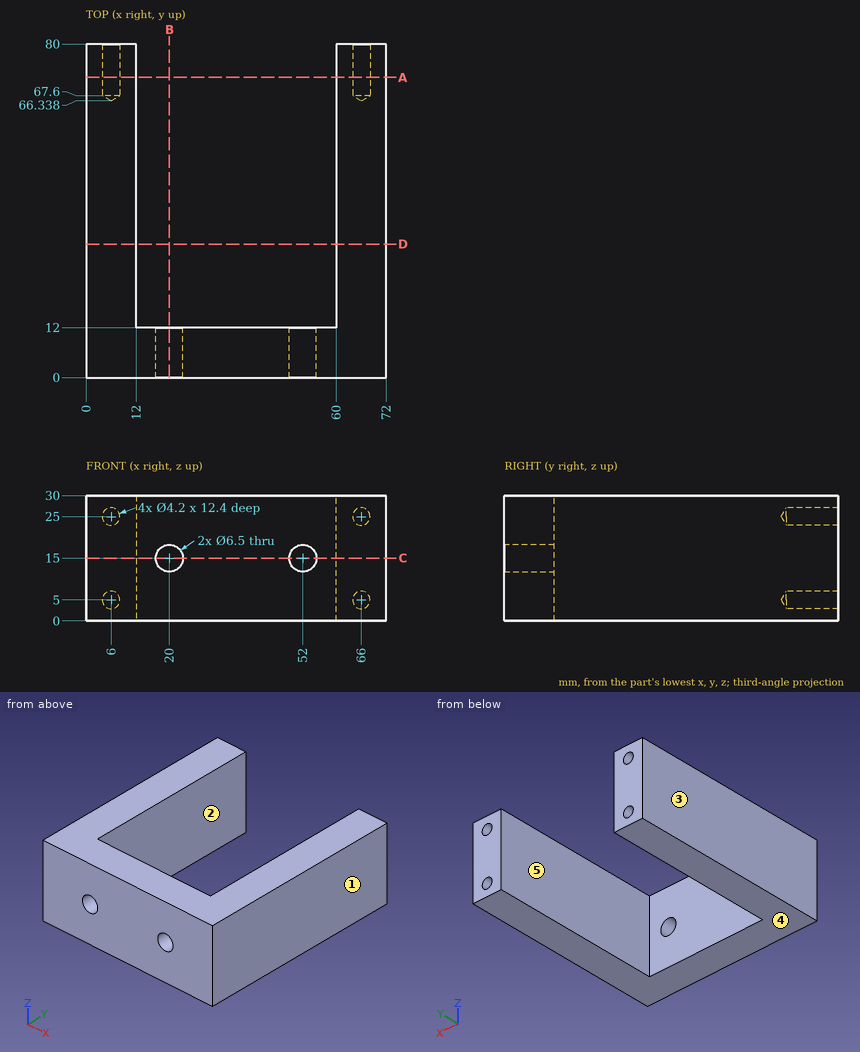
The drawing under review shows one solid part. Ordinate dimensions are in mm from its lowest x, y, z. A direction names the side the tool comes from. Coordinates: 2 decimals unless noted, no trailing zeros. Write each loop counter-clockwise with the first axis right and the second up, starting at its lowest first coordinate (ties: lowest second). Pieces come first, ordered by that corner, then holes. Notation, with made-up numbers: (-31.5, -14) - (11.5, -14) arc R30 cw to (11.5, 15) - close; hole circle Ø9 at (84.25, 38). An arc over 180 degrees is marked (long way). Answer as CSV lines item,"result".
(1) We need section A-A (y = 72). Give the boundary of the cut face in (x, z).
Data:
outline,"(0, 0) - (12, 0) - (12, 30) - (0, 30) - close; (60, 0) - (72, 0) - (72, 30) - (60, 30) - close; hole circle Ø4.2 at (6, 5); hole circle Ø4.2 at (6, 25); hole circle Ø4.2 at (66, 5); hole circle Ø4.2 at (66, 25)"
(2) We need section B-B (x = 20). Give the boundary of the cut face in (y, z).
Data:
outline,"(0, 0) - (12, 0) - (12, 11.75) - (0, 11.75) - close; (0, 18.25) - (12, 18.25) - (12, 30) - (0, 30) - close"
(3) Tool access review of the marked faces 1 and 2: name each direction out of +Z, -Z, +X, -X, +Y, -Y from which nothing blocks a thin tool from reaching the whole face with its end or side.
Data:
face 1,"+Z, -Z, +X, +Y, -Y"
face 2,"+Z, -Z, +Y"
(4) Mouldability with a two-part tool opening along X and no side actions: class the marked faces 3, 4 and 5 as pulls with the +X half, pulls with the -X half, needs draft (parallel to the pull), parting line crosses it, or undercut.
Data:
face 3,"pulls with the -X half"
face 4,"needs draft"
face 5,"undercut"
(5) We need section D-D (y = 32). Give the boundary of the cut face in (x, z).
Data:
outline,"(0, 0) - (12, 0) - (12, 30) - (0, 30) - close; (60, 0) - (72, 0) - (72, 30) - (60, 30) - close"
(6) Clearance check with flat-ended pins moving along their axes: pin 1 Ø2.5 at (x, z) = (6, 5) entering from +Y; pin 2 Ø4 at (x, z) = (21.5, 3.5) entering from +Y; pin 3 Ø4 at (x, z) = (52, 15) entering from +Y. State where each tip first meets the part, or that it passes through.
Data:
pin 1,"stops at y = 67.09"
pin 2,"stops at y = 12"
pin 3,"passes through"
(7) For line 1 along X through (y, z) = (6.25, 15); line 2 along X through (y, z) = (72, 5); line 3 along Z through (x, y) = (6, 71.25), list the stretches that pass through material, from the lowest coordinate up. Write a range as [from, to].
Data:
line 1,"x = [0, 16.75], [23.25, 48.75], [55.25, 72]"
line 2,"x = [0, 3.9], [8.1, 12], [60, 63.9], [68.1, 72]"
line 3,"z = [0, 2.9], [7.1, 22.9], [27.1, 30]"
(8) We need section C-C (z = 15). Give the boundary of the cut face in (x, y), plus the area to 3 significant figures.
Data:
outline,"(0, 0) - (16.75, 0) - (16.75, 12) - (12, 12) - (12, 80) - (0, 80) - close; (23.25, 0) - (48.75, 0) - (48.75, 12) - (23.25, 12) - close; (55.25, 0) - (72, 0) - (72, 80) - (60, 80) - (60, 12) - (55.25, 12) - close"
area,"2,340 mm2"
